The drawing under review shows one solid part. Ordinate dimensions are in mm from its lowest x, y, z. Coordinates: 2 decimals unless noted, no trailing zeros. Order: outer loops, then holes, each group sorted by start corner. A loop starts at its lowest first (then second) coordinate and runs counter-clockwise, first axis right, second up. Notation, with made-up numbers: (-9.75, 43) - (23.25, 43) arc R19 ccw to (23.25, 66) - close; hole circle Ø3 at (-34, -5.75). An arc over 180 degrees is marked (long way). Answer in a Markdown table with one row per item.
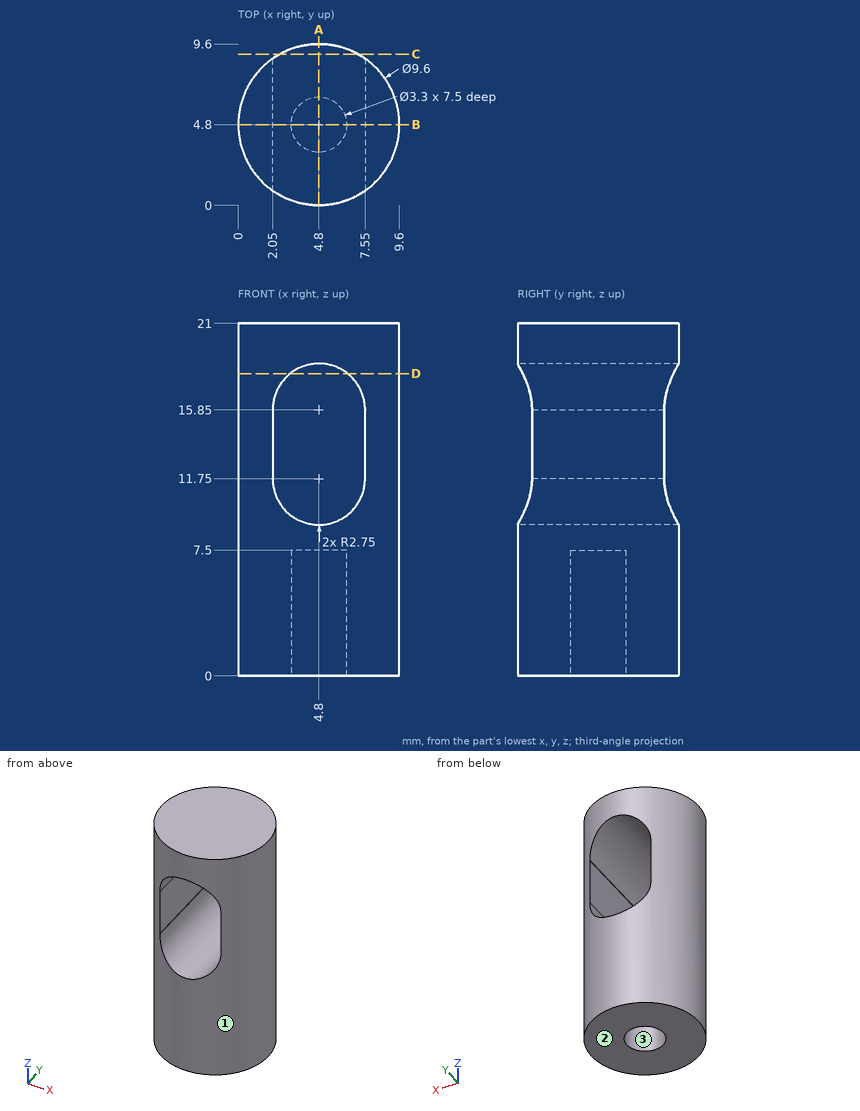
Item 1: Clearance check with flat-ended pins moving along their axes: pin 1 Ø2 at (x, z) = (4.5, 3) entering from -Y; pin 2 Ø1 at (x, y) = (5, 4.5) entering from -Z. State where each tip first meets the part, or that it passes through.
Check values:
| item | result |
|---|---|
| pin 1 | y = 0 |
| pin 2 | z = 7.5 |
Item 2: We need section C-C, the plane y = 9. Write out the cut boundary in (x, z).
Check values:
| item | result |
|---|---|
| outline | (2.48, 0) - (7.12, 0) - (7.12, 10.28) arc R2.75 cw to (2.48, 10.28) - close; (2.48, 17.32) arc R2.75 cw to (7.12, 17.32) - (7.12, 21) - (2.48, 21) - close |
Item 3: We need section D-D, the plane z = 18. Write out the cut boundary in (x, y) (1 decimal).
Check values:
| item | result |
|---|---|
| outline | (3.1, 0.3) - (3.1, 9.3) arc R4.8 ccw to start; (6.5, 0.3) arc R4.8 ccw to (6.5, 9.3) - close |
Item 4: Mouldability with a two-part tool opening along X and no side actions: class the marked faces 1, 2 and 3 as +X half, -X half, draft (parallel to the pull), parting line (faces both ways), or undercut.
Check values:
| item | result |
|---|---|
| face 1 | parting line |
| face 2 | draft |
| face 3 | undercut |
Item 5: We need section B-B, the plane y = 4.8. Write out the cut boundary in (x, z).
Check values:
| item | result |
|---|---|
| outline | (0, 0) - (3.15, 0) - (3.15, 7.5) - (6.45, 7.5) - (6.45, 0) - (9.6, 0) - (9.6, 21) - (0, 21) - close; hole (2.05, 11.78) arc R2.75 ccw (long way) to (7.55, 11.75) - (7.55, 15.81) arc R2.75 ccw (long way) to (2.05, 15.85) - close |
Item 6: We need section A-A, the plane x = 4.8. Write out the cut boundary in (y, z).
Check values:
| item | result |
|---|---|
| outline | (0, 0) - (3.15, 0) - (3.15, 7.5) - (6.45, 7.5) - (6.45, 0) - (9.6, 0) - (9.6, 9) - (0, 9) - close; (0, 18.6) - (9.6, 18.6) - (9.6, 21) - (0, 21) - close |
Item 7: To check wall thickness, follow line 1 (Y direction, x = 4.8, z = 2); line 2 (Z direction, x = 5.75, y = 4.5); line 3 (X direction, y = 6, z = 12.5). State the ranges of each line that lie inside material, in increasing order. Write a range as from..to.
Check values:
| item | result |
|---|---|
| line 1 | 0..3.15, 6.45..9.6 |
| line 2 | 7.5..9.17, 18.43..21 |
| line 3 | 0.15..2.05, 7.55..9.45 |
